Autodesk Inventor part; units mm, degrees
ref_plane "YZ Plane" through (0, 0, 0) normal (1, 0, 0) x (0, 1, 0)
ref_plane "XZ Plane" through (0, 0, 0) normal (0, 1, 0) x (-1, 0, 0)
ref_plane "XY Plane" through (0, 0, 0) normal (0, 0, 1) x (1, 0, 0)
sketch "Esboço1" plane through (0, 0, 0) normal (0, 0, 1) x (-1, 0, 0)
  circle A0 centre (0, 0) radius 25
  dimension "d0" = 50
extrude "Extrusão1" add sketch "Esboço1" along normal mid plane 5
sketch "Esboço2" plane through (0, 0, 0) normal (0, 0, -1) x (1, 0, 0)
  circle A0 centre (0, 0) radius 20
  dimension "d3" = 40
extrude "Extrusão2" add sketch "Esboço2" along normal blind 156
sketch "Esboço3" plane through (0, 0, 0) normal (0, 0, 1) x (1, 0, 0)
  circle A0 centre (0, 0) radius 17.5
  dimension "d6" = 35
extrude "Extrusão3" add sketch "Esboço3" along normal blind 29
chamfer "Chanfro1" distance 1 angle 45 1 edges at (-20, 0, -156)
chamfer "Chanfro2" distance 1 angle 45 3 edges at (25, 0, -2.5) (25, 0, 2.5) (-17.5, 0, 29)
properties material "Liga de aço"
Design review of the part built by this model. Coordinates are the model's own, in mm. A direction names the side the tool comes from. Coordinates: 2 decimals unless noted, no trailing zeros. Loops run counter-clockwise (first coordinate to the right, second up) from the corner with the lowest first, then second, coordinate; pieces in that order, holes last.
Item 1: For faces 1 (the flat face through (-2, 18, 2.5)), 2 (the flat face through (0, 0, 29)), 3 (the flat face through (5, -20, -2.5)), list the 3-axis set-ups (+Z, -Z, +X, -X, +Y, -Y) from which the entire face can be reached by the end or side of a thin tool; tool diameter is ignored.
Completed:
face 1: +Z
face 2: +Z, +X, -X, +Y, -Y
face 3: -Z
Item 2: Clearance check with flat-ended pins moving along their axes: pin 1 (10 mm diameter, centred on x = 17, z = -111.5, fed in from +Y); pin 2 (2 mm diameter, centred on x = -0.5, z = -33.5, fed in from -Y); pin 3 (1.5 mm diameter, centred on x = 4.5, y = -19.5, fed in from -Z). State where each tip first meets the part, or that it passes through.
Completed:
pin 1: stops at y = 16
pin 2: stops at y = -20
pin 3: stops at z = -155.74
Item 3: Add section C-C (z = -50). Write out the cut boundary in (x, y).
Completed:
outline: circle Ø40 at (0, 0)
Item 4: Wall thickness on L1, parallel to Z at x = 17, y = -14.5; L2, parallel to Z at x = 19, y = 1; L3, parallel to Y at x = 15.5, z = -48: over which ranges is each line inside the solid? List them lowest first.
Completed:
L1: z = -2.5 to 2.5
L2: z = -155.97 to 2.5
L3: y = -12.64 to 12.64
Item 5: Add section A-A (y = 0). Write out the cut boundary in (x, z), and give its area (3 significant figures).
Completed:
outline: (-25, -1.5) - (-24, -2.5) - (-20, -2.5) - (-20, -155) - (-19, -156) - (19, -156) - (20, -155) - (20, -2.5) - (24, -2.5) - (25, -1.5) - (25, 1.5) - (24, 2.5) - (17.5, 2.5) - (17.5, 28) - (16.5, 29) - (-16.5, 29) - (-17.5, 28) - (-17.5, 2.5) - (-24, 2.5) - (-25, 1.5) - close
area: 7,310 mm2
